from build123d import *
from build123d.topology import SkipClean

# Parameters (mm, degrees)
BOSS_EXTRUDE1_DEPTH = 42.000000074
BOSS_EXTRUDE4_START = 2.000000064
BOSS_EXTRUDE4_DEPTH = 2.000000064


with BuildPart() as part:
    # Sketch1 → Boss-Extrude1 (new body)
    with BuildSketch(Plane(origin=(0, 0, 0), x_dir=(0, 0, -1), z_dir=(1, 0, 0))):
        with BuildLine():
            Line((-95.033966152, 0.044726877), (-92.443504117, 0.003255065))
            ThreePointArc((-92.443504117, 0.003255065), (-24.995368101, 141.699621751), (42.445929187, 0))
            Line((42.445929187, 0), (45.004045198, 0))
            ThreePointArc((45.004045198, 0), (-24.96907126, 143.699617306), (-95.033966152, 0.044726877))
        make_face()
    extrude(amount=-BOSS_EXTRUDE1_DEPTH)

    # Sketch2 → Boss-Extrude4 (add)
    with SkipClean():  # the faces are left unmerged after this step: merging them gives an invalid solid
        with BuildSketch(Plane(origin=(0, 0, 0), x_dir=(0, 0, -1), z_dir=(1, 0, 0)).offset(BOSS_EXTRUDE4_START)):
            with BuildLine():
                Line((-122.000000064, 0), (-120, 0))
                Line((-120, 0), (-95.033966152, 0.044726877))
                ThreePointArc((-95.033966152, 0.044726877), (-113.897460426, 54.828495951), (-94.998383349, 109.6))
                Line((-94.998383349, 109.6), (-120, 109.6))
                Line((-120, 109.6), (-122.000000064, 109.6))
                Line((-122.000000064, 109.6), (-122.000000064, 0))
            make_face()
            with BuildLine():
                ThreePointArc((-95.033966152, 0.044726877), (-24.937426484, 143.699601567), (44.965014594, -0.049821483))
                Line((44.965014594, -0.049821483), (42.445929187, 0))
                ThreePointArc((42.445929187, 0), (-24.995368101, 141.699621751), (-92.443504117, 0.003255065))
                Line((-92.443504117, 0.003255065), (-95.033966152, 0.044726877))
            make_face()
            with BuildLine():
                Line((50, 109.6), (45.003453118, 109.6))
                ThreePointArc((45.003453118, 109.6), (63.902529422, 54.768457316), (44.965014594, -0.049821483))
                Line((44.965014594, -0.049821483), (160, 0))
                Line((160, 0), (162.000000064, 0))
                Line((162.000000064, 0), (162.000000064, 109.6))
                Line((162.000000064, 109.6), (160, 109.6))
                Line((160, 109.6), (50, 109.6))
            make_face()
        extrude(amount=-BOSS_EXTRUDE4_DEPTH)


solid = part.part
The model under review builds one solid part; all positions refer to its coordinate system, in mm. A direction names the side the tool comes from. Coordinates: 2 decimals unless noted, no trailing zeros. Loops run counter-clockwise (first coordinate to the right, second up) from the corner with the lowest first, then second, coordinate; pieces in that order, holes last. Notation, with made-up numbers: (31.25, 32) -> (59.25, 32) arc R27 cw to (59.25, 51) -> close; hole circle Ø5 at (-10, 46). An arc over 180 degrees is marked (long way). Use a Markdown table: item, result. Add a question column.
1. Add section C-C on z = 84.5. Write out the cut boundary in (x, y), plus the area to 3 significant figures.
2. To check wall thickness, follow line 1 (Z direction, x = -2, y = 53); line 2 (Z direction, x = -7, y = 93); line 3 (Y direction, x = -18.5, z = -48). State the ranges of each line that lie inside material, in increasing order.
3. Clearance check with flat-ended pins moving along their axes: pin 1 Ø2 at (x, y) = (-32, 79.5) entering from +Z; pin 2 Ø0.6 at (x, z) = (1.5, 115) entering from +Y; pin 3 Ø0.8 at (x, z) = (-19.5, -43.5) entering from -Y. State where each tip first meets the part, or that it passes through.
4. Machinability: for faces 1 (the face through (0, 56, 115)), 2 (the face through (-42, 136, -8)), which of the approach directions +Z, -Z, +X, -X, +Y, -Y give a long, thin tool a straight path to every point of the face, cutting with its end or side? Answer none if there is none.
5. Add section D-D on y = 117.5. Write out the cut boundary in (x, z).
6. Add section B-B on x = -13.5. Write out the cut boundary in (y, z), plus the area to 3 significant figures.
7. Add section A-A on y = 40.5. Write out the cut boundary in (x, z), plus the area to 3 significant figures.
Returned:
| question | item | result |
|---|---|---|
| 1 | outline | (-42, 118.13) -> (2, 118.13) -> (2, 120.85) -> (-42, 120.85) -> close |
| 1 | area | 120 mm² |
| 2 | line 1 | z = -63.88 to -61.88, 111.88 to 113.88 |
| 2 | line 2 | z = -55.28 to -53.06, 103.05 to 105.27 |
| 2 | line 3 | y = 4.06 to 7.65, 101.95 to 105.54 |
| 3 | pin 1 | stops at z = 110.68 |
| 3 | pin 2 | stops at y = 109.6 |
| 3 | pin 3 | stops at y = 0 |
| 4 | face 1 | +Z, -X |
| 4 | face 2 | +Z, -Z, -X, +Y, -Y |
| 5 | outline | (-42, -38.03) -> (2, -38.03) -> (2, -35.17) -> (-42, -35.17) -> close; (-42, 85.17) -> (2, 85.17) -> (2, 88.02) -> (-42, 88.02) -> close |
| 6 | outline | (0, -45) arc R88.9 ccw (long way) to (0.04, 95.03) -> (0, 92.44) arc R86.9 cw (long way) to (0, -42.45) -> close |
| 6 | area | 789 mm² |
| 7 | outline | (-42, -62.74) -> (0, -62.74) -> (0, -162) -> (2, -162) -> (2, -60.72) -> (-42, -60.72) -> close; (-42, 110.71) -> (2, 110.71) -> (2, 122) -> (0, 122) -> (0, 112.74) -> (-42, 112.74) -> close |
| 7 | area | 395 mm² |
